Could you check a few things on this model? Use its own coordinates, in mm. A direction names the side the tool comes from. Coordinates: 2 decimals unless noted, no trailing zeros. Write each loop counter-clockwise with the first axis right and the second up, starting at its lowest first coordinate (ties: lowest second). Pieces come first, ordered by that corner, then holes. Notation, with made-up numbers: (78.5, 8) - (135.5, 8) arc R27 cw to (135.5, 25) - close; hole circle Ø8 at (-27.75, 80.25). An arc over 180 degrees is marked (long way). Answer as a JSON object with one key per item and string values. Group by question number.
1) Will these pins go through, and if not, where does the flat tip stop? pin 1 Ø5 at (x, y) = (10.825, 0) entering from +Z; pin 2 Ø1 at (y, z) = (0, 0.5) entering from +X; pin 3 Ø0.6 at (x, y) = (13.5, -1) entering from -Z; pin 4 Ø1.5 at (x, z) = (30.5, 4.5) entering from +Y.
2) If we section it at D-D (z = 7): Write out the boundary of the cut face in (x, y) (3 decimals), plus the area to 3 significant figures.
3) If we section it at A-A (z = 4.5): Write out the boundary of the cut face in (x, y) (3 decimals), plus the area to 3 significant figures.
4) On a 3-axis mill with a long thin cutter (end or side, diameter ignored), from which of +Z, -Z, +X, -X, +Y, -Y can I reach the whole of each face in a straight line? I mean faces 1 (the flat face through (13.3, 0, 2.5)), 2 (the flat face through (24.02, 0, 0)), 3 (the cylindrical face through (11.838, -4.564, 6.282)). Say none if no direction works.
5) Please list where these lines run through material, in increasing order: line 1 along Y through (x, z) = (11.25, 0); line 2 along Z through (x, y) = (3, 0); line 3 along X through (y, z) = (0, 7.25).
6) If we section it at B-B (x = 8): Write out the boundary of the cut face in (y, z).
7) We'd pull the mould along Z, two halves only. Please class faces 4 (the flat face through (9.85, 2.14, 8.5)), 5 (the flat face through (40.32, -2.4, 2.5)), 6 (the cylindrical face through (6.9, 0.11, -3.05)): released by +Z, released by -Z, zero draft, split by the parting line, or undercut.
8) If we section it at C-C (x = 23): Write out the boundary of the cut face in (y, z).
```python
from build123d import *

# Parameters (mm, degrees)
SKETCH1_R           = 5.5
BOSS_EXTRUDE1_DEPTH = 14
SKETCH2_R           = 5.5
BOSS_EXTRUDE2_DEPTH = 13.52
SKETCH3_R           = 5.5
BOSS_EXTRUDE3_DEPTH = 12.8
SKETCH4_R           = 1.05
CUT_EXTRUDE1_DEPTH  = 3.5
SKETCH5_R           = 4.675
SKETCH5_R_2         = 2.175
BOSS_EXTRUDE4_DEPTH = 6
SKETCH5_2_R         = 2.175
CUT_EXTRUDE2_DEPTH  = 42.472308963


with BuildPart() as part:
    # Sketch1 → Boss-Extrude1 (new body)
    with BuildSketch(Plane.YZ):
        with Locations(Location((0, 0, 0), (0, 0, 270))):
            Circle(SKETCH1_R)
        with BuildLine():
            Line((-1.747140521, 2.5), (1.747140521, 2.5))
            ThreePointArc((1.747140521, 2.5), (0, -3.05), (-1.747140521, 2.5))
        make_face(mode=Mode.SUBTRACT)
    extrude(amount=BOSS_EXTRUDE1_DEPTH)

    # Sketch2 → Boss-Extrude2 (add)
    with BuildSketch(Plane.YZ.offset(14)):
        with Locations(Location((0, 0, 0), (0, 0, 270))):
            Circle(SKETCH2_R)
    extrude(amount=BOSS_EXTRUDE2_DEPTH)

    # Sketch3 → Boss-Extrude3 (add)
    with BuildSketch(Plane.YZ.offset(27.52)):
        with Locations(Location((0, 0, 0), (0, 0, 270))):
            Circle(SKETCH3_R)
        with BuildLine():
            ThreePointArc((-1.322019746, -2.893008891), (-1.318956528, -2.868853063), (-1.317084788, -2.844575833))
            ThreePointArc((-1.317084788, -2.844575833), (-1.543809469, -2.402214423), (-2.040380396, -2.37974197))
            ThreePointArc((-2.040380396, -2.37974197), (-2.061686193, -2.391529691), (-2.0823866, -2.404350785))
            ThreePointArc((-2.0823866, -2.404350785), (-2.380259348, -2.555545236), (-2.703854763, -2.638454478))
            ThreePointArc((-2.703854763, -2.638454478), (-2.855120731, -2.473976197), (-2.996397469, -2.300842198))
            ThreePointArc((-2.996397469, -2.300842198), (-2.868279694, -1.992339732), (-2.676232473, -1.719016114))
            ThreePointArc((-2.676232473, -1.719016114), (-2.660595904, -1.700351039), (-2.645896034, -1.680939672))
            ThreePointArc((-2.645896034, -1.680939672), (-2.597470339, -1.186224957), (-3.003062861, -0.898853414))
            ThreePointArc((-3.003062861, -0.898853414), (-3.02735936, -0.897251093), (-3.051705258, -0.896845399))
            ThreePointArc((-3.051705258, -0.896845399), (-3.384033651, -0.862996099), (-3.701083558, -0.757794901))
            ThreePointArc((-3.701083558, -0.757794901), (-3.739412915, -0.537646409), (-3.764659163, -0.315616851))
            ThreePointArc((-3.764659163, -0.315616851), (-3.490090608, -0.12535376), (-3.1807603, 0.000752133))
            ThreePointArc((-3.1807603, 0.000752133), (-3.157514879, 0.008000426), (-3.134653985, 0.016382957))
            ThreePointArc((-3.134653985, 0.016382957), (-2.82645273, 0.406382552), (-3.012294086, 0.86741475))
            ThreePointArc((-3.012294086, 0.86741475), (-3.031867321, 0.881898388), (-3.052129059, 0.895402065))
            ThreePointArc((-3.052129059, 0.895402065), (-3.31340118, 1.103548202), (-3.523244473, 1.363459202))
            ThreePointArc((-3.523244473, 1.363459202), (-3.43646792, 1.569382314), (-3.337668173, 1.769814617))
            ThreePointArc((-3.337668173, 1.769814617), (-3.003822413, 1.781431146), (-2.675419206, 1.720281583))
            ThreePointArc((-2.675419206, 1.720281583), (-2.65194519, 1.713811812), (-2.628181444, 1.708504114))
            ThreePointArc((-2.628181444, 1.708504114), (-2.158056349, 1.869966471), (-2.065143222, 2.35828486))
            ThreePointArc((-2.065143222, 2.35828486), (-2.07377883, 2.381051361), (-2.083523449, 2.4033657))
            ThreePointArc((-2.083523449, 2.4033657), (-2.190787246, 2.719723746), (-2.226800162, 3.051824643))
            ThreePointArc((-2.226800162, 3.051824643), (-2.042468641, 3.178143241), (-1.850991121, 3.293342448))
            ThreePointArc((-1.850991121, 3.293342448), (-1.563861826, 3.12262425), (-1.320651417, 2.893633786))
            ThreePointArc((-1.320651417, 2.893633786), (-1.304401641, 2.875500057), (-1.287279864, 2.858187286))
            ThreePointArc((-1.287279864, 2.858187286), (-0.804492326, 2.739849249), (-0.462323977, 3.100416189))
            ThreePointArc((-0.462323977, 3.100416189), (-0.457280213, 3.124237351), (-0.453413865, 3.148277707))
            ThreePointArc((-0.453413865, 3.148277707), (-0.372613841, 3.472406218), (-0.223362534, 3.771257322))
            ThreePointArc((-0.223362534, 3.771257322), (-0.111730141, 3.776213578), (0, 3.777866145))
            ThreePointArc((0, 3.777866145), (0.111730141, 3.776213578), (0.223362534, 3.771257322))
            ThreePointArc((0.223362534, 3.771257322), (0.372613841, 3.472406218), (0.453413865, 3.148277707))
            ThreePointArc((0.453413865, 3.148277707), (0.457280213, 3.124237351), (0.462323977, 3.100416189))
            ThreePointArc((0.462323977, 3.100416189), (0.804492326, 2.739849249), (1.287279864, 2.858187286))
            ThreePointArc((1.287279864, 2.858187286), (1.304401641, 2.875500057), (1.320651417, 2.893633786))
            ThreePointArc((1.320651417, 2.893633786), (1.563861826, 3.12262425), (1.850991121, 3.293342448))
            ThreePointArc((1.850991121, 3.293342448), (2.042468641, 3.178143241), (2.226800162, 3.051824643))
            ThreePointArc((2.226800162, 3.051824643), (2.190787246, 2.719723746), (2.083523449, 2.4033657))
            ThreePointArc((2.083523449, 2.4033657), (2.07377883, 2.381051361), (2.065143222, 2.35828486))
            ThreePointArc((2.065143222, 2.35828486), (2.158056349, 1.869966471), (2.628181444, 1.708504114))
            ThreePointArc((2.628181444, 1.708504114), (2.65194519, 1.713811812), (2.675419206, 1.720281583))
            ThreePointArc((2.675419206, 1.720281583), (3.003822413, 1.781431146), (3.337668173, 1.769814617))
            ThreePointArc((3.337668173, 1.769814617), (3.43646792, 1.569382314), (3.523244473, 1.363459202))
            ThreePointArc((3.523244473, 1.363459202), (3.31340118, 1.103548202), (3.052129059, 0.895402065))
            ThreePointArc((3.052129059, 0.895402065), (3.031867321, 0.881898388), (3.012294086, 0.86741475))
            ThreePointArc((3.012294086, 0.86741475), (2.82645273, 0.406382552), (3.134653985, 0.016382957))
            ThreePointArc((3.134653985, 0.016382957), (3.157514879, 0.008000426), (3.1807603, 0.000752133))
            ThreePointArc((3.1807603, 0.000752133), (3.490090608, -0.12535376), (3.764659163, -0.315616851))
            ThreePointArc((3.764659163, -0.315616851), (3.739412915, -0.537646409), (3.701083558, -0.757794901))
            ThreePointArc((3.701083558, -0.757794901), (3.384033651, -0.862996099), (3.051705258, -0.896845399))
            ThreePointArc((3.051705258, -0.896845399), (3.02735936, -0.897251093), (3.003062861, -0.898853414))
            ThreePointArc((3.003062861, -0.898853414), (2.597470339, -1.186224957), (2.645896034, -1.680939672))
            ThreePointArc((2.645896034, -1.680939672), (2.660595904, -1.700351039), (2.676232473, -1.719016114))
            ThreePointArc((2.676232473, -1.719016114), (2.868279694, -1.992339732), (2.996397469, -2.300842198))
            ThreePointArc((2.996397469, -2.300842198), (2.855120731, -2.473976197), (2.703854763, -2.638454478))
            ThreePointArc((2.703854763, -2.638454478), (2.380259349, -2.555545235), (2.082386604, -2.404350784))
            ThreePointArc((2.082386604, -2.404350784), (2.061686196, -2.39152969), (2.0403804, -2.379741969))
            ThreePointArc((2.0403804, -2.379741969), (1.54380947, -2.402214422), (1.317084788, -2.844575834))
            ThreePointArc((1.317084788, -2.844575834), (1.318956528, -2.868853064), (1.322019746, -2.893008892))
            ThreePointArc((1.322019746, -2.893008892), (1.335810244, -3.226771918), (1.27680075, -3.555566405))
            ThreePointArc((1.27680075, -3.555566405), (1.064347889, -3.624836022), (0.848171186, -3.6814234))
            ThreePointArc((0.848171186, -3.6814234), (0.62076952, -3.436726817), (0.45192491, -3.148491786))
            ThreePointArc((0.45192491, -3.148491786), (0.441442226, -3.12651451), (0.429891573, -3.105079266))
            ThreePointArc((0.429891573, -3.105079266), (0, -2.855517783), (-0.429891573, -3.105079265))
            ThreePointArc((-0.429891573, -3.105079265), (-0.441442226, -3.12651451), (-0.45192491, -3.148491786))
            ThreePointArc((-0.45192491, -3.148491786), (-0.62076952, -3.436726817), (-0.848171186, -3.6814234))
            ThreePointArc((-0.848171186, -3.6814234), (-1.064347889, -3.624836022), (-1.27680075, -3.555566405))
            ThreePointArc((-1.27680075, -3.555566405), (-1.335810244, -3.226771917), (-1.322019746, -2.893008891))
        make_face(mode=Mode.SUBTRACT)
    extrude(amount=BOSS_EXTRUDE3_DEPTH)

    # Sketch4 → Cut-Extrude1 (cut)
    with BuildSketch(Plane.YZ.offset(27.52)):
        with Locations(Location((0, 0, 0), (0, 0, 270))):
            Circle(SKETCH4_R)
    extrude(amount=-CUT_EXTRUDE1_DEPTH, mode=Mode.SUBTRACT)

    # Sketch5 → Boss-Extrude4 (add)
    with BuildSketch(Plane(origin=(0, 0, 2.5), x_dir=(-1, 0, 0), z_dir=(0, 0, -1))):
        with Locations((-10.825, 0)):
            Circle(SKETCH5_R)
        with Locations((-10.825, 0)):
            Circle(SKETCH5_R_2, mode=Mode.SUBTRACT)
    extrude(amount=-BOSS_EXTRUDE4_DEPTH)

    # Sketch5_2 → Cut-Extrude2 (cut, through all)
    with BuildSketch(Plane(origin=(0, 0, 2.5), x_dir=(-1, 0, 0), z_dir=(0, 0, -1))):
        with Locations((-10.825, 0)):
            Circle(SKETCH5_2_R)
    extrude(amount=-CUT_EXTRUDE2_DEPTH, mode=Mode.SUBTRACT)


solid = part.part
```
Here are the results:
{
 "1": {"pin 1": "stops at z = 8.5", "pin 2": "stops at x = 24.02", "pin 3": "stops at z = -5.46", "pin 4": "stops at y = 4.02"},
 "2": {"outline": "circle Ø9.35 at (10.825, 0); hole circle Ø4.35 at (10.825, 0)", "area": "53.8 mm²"},
 "3": {"outline": "(0, -3.162) - (7.382, -3.162) arc R4.675 ccw to (14.268, -3.162) - (40.32, -3.162) - (40.32, 3.162) - (14.268, 3.162) arc R4.675 ccw to (7.382, 3.162) - (0, 3.162) - close; hole circle Ø4.35 at (10.825, 0)", "area": "255 mm²"},
 "4": {"face 1": "-X", "face 2": "+X", "face 3": "+Z"},
 "5": {"line 1": "y = -5.5 to -3.05, 3.05 to 5.5", "line 2": "z = -5.5 to -3.05, 2.5 to 5.5", "line 3": "x = 6.15 to 8.65, 13 to 15.5"},
 "6": {"outline": "(-3.72, 4.05) arc R5.5 ccw (long way) to (3.72, 4.05) - (3.72, 8.5) - (-3.72, 8.5) - close; hole (-1.75, 2.5) arc R3.05 ccw (long way) to (1.75, 2.5) - close"},
 "7": {"face 4": "released by +Z", "face 5": "zero draft", "face 6": "undercut"},
 "8": {"outline": "circle Ø11 at (0, 0)"}
}
